Geometry: final body of the model. Coordinates: model frame, mm. A direction names the side the tool comes from. Give positions to 0.01 mm unless a question says otherwise; leave off trailing zeros. Order: outer loops, then holes, each group sorted by start corner. A loop starts at its lowest first (then second) coordinate and runs counter-clockwise, first axis right, second up. Notation, with made-up numbers: (59.5, 45.25) -> (93.5, 45.25) arc R26 ccw to (93.5, 80.25) -> close; hole circle Ø2 at (-21, 81). An arc over 180 degrees is marked (long way). One line per item, written item: value. Start each with the question number.
```python
from build123d import *

# Parameters (mm, degrees)
SKETCH17_R                     = 3.4
SKETCH17_W                     = 3.75
SKETCH17_H                     = 3.75
T_SLOT_PROFILES_3030_2_1_DEPTH = 400


with BuildPart() as part:
    # Sketch17 → T-slot profiles 3030_2(1) (new body)
    with BuildSketch(Plane(origin=(0, 0, 0), x_dir=(0, 0, -1), z_dir=(1, 0, 0))):
        with BuildLine():
            Line((-4.07, 5.6), (4.07, 5.6))
            Line((4.07, 5.6), (8.25, 9.78))
            Line((8.25, 9.78), (8.25, 13))
            Line((8.25, 13), (4.07, 13))
            Line((4.07, 13), (4.07, 15))
            Line((4.07, 15), (12.5, 15))
            ThreePointArc((12.5, 15), (14.267766953, 14.267766953), (15, 12.5))
            Line((15, 12.5), (15, 4.07))
            Line((15, 4.07), (13, 4.07))
            Line((13, 4.07), (13, 8.25))
            Line((13, 8.25), (9.78, 8.25))
            Line((9.78, 8.25), (5.6, 4.07))
            Line((5.6, 4.07), (5.6, -4.07))
            Line((5.6, -4.07), (9.78, -8.25))
            Line((9.78, -8.25), (13, -8.25))
            Line((13, -8.25), (13, -4.07))
            Line((13, -4.07), (15, -4.07))
            Line((15, -4.07), (15, -12.5))
            ThreePointArc((15, -12.5), (14.267766953, -14.267766953), (12.5, -15))
            Line((12.5, -15), (4.07, -15))
            Line((4.07, -15), (4.07, -13))
            Line((4.07, -13), (8.25, -13))
            Line((8.25, -13), (8.25, -9.78))
            Line((8.25, -9.78), (4.07, -5.6))
            Line((4.07, -5.6), (-4.07, -5.6))
            Line((-4.07, -5.6), (-8.25, -9.78))
            Line((-8.25, -9.78), (-8.25, -13))
            Line((-8.25, -13), (-4.07, -13))
            Line((-4.07, -13), (-4.07, -15))
            Line((-4.07, -15), (-12.5, -15))
            ThreePointArc((-12.5, -15), (-14.267766953, -14.267766953), (-15, -12.5))
            Line((-15, -12.5), (-15, -4.07))
            Line((-15, -4.07), (-13, -4.07))
            Line((-13, -4.07), (-13, -8.25))
            Line((-13, -8.25), (-9.78, -8.25))
            Line((-9.78, -8.25), (-5.6, -4.07))
            Line((-5.6, -4.07), (-5.6, 4.07))
            Line((-5.6, 4.07), (-9.78, 8.25))
            Line((-9.78, 8.25), (-13, 8.25))
            Line((-13, 8.25), (-13, 4.07))
            Line((-13, 4.07), (-15, 4.07))
            Line((-15, 4.07), (-15, 12.5))
            ThreePointArc((-15, 12.5), (-14.267766953, 14.267766953), (-12.5, 15))
            Line((-12.5, 15), (-4.07, 15))
            Line((-4.07, 15), (-4.07, 13))
            Line((-4.07, 13), (-8.25, 13))
            Line((-8.25, 13), (-8.25, 9.78))
            Line((-8.25, 9.78), (-4.07, 5.6))
        make_face()
        Circle(SKETCH17_R, mode=Mode.SUBTRACT)
        with Locations((11.625, 11.625)):
            Rectangle(SKETCH17_W, SKETCH17_H, mode=Mode.SUBTRACT)
        with Locations((11.625, -11.625)):
            Rectangle(SKETCH17_W, SKETCH17_H, mode=Mode.SUBTRACT)
        with Locations((-11.625, 11.625)):
            Rectangle(SKETCH17_W, SKETCH17_H, mode=Mode.SUBTRACT)
        with Locations((-11.625, -11.625)):
            Rectangle(SKETCH17_W, SKETCH17_H, mode=Mode.SUBTRACT)
    extrude(amount=T_SLOT_PROFILES_3030_2_1_DEPTH)


solid = part.part
```
1. Draft query along Y for faces 6 (the flat face through (197, -15, 8)), 7 (the flat face through (400, -3, 2)), 8 (the flat face through (197, 0, 5.6)). Return one class per face: pulls with the +Y half, pulls with the -Y half, needs draft (parallel to the pull), parting line crosses it, or undercut.
2. Cut plane C-C, the plane x = 92. State how many separate pieces and enclosed holes the cut face has, then the cut area to 3 significant figures.
3. Cut plane A-A, the plane z = 0. Return loops of the section in (x, y), then the cut area to 3 significant figures.
4. Pin query (flat end, axial travel): P1, Ø0.6, axis at x = 110, z = -14, coming from the +Y side; P2, Ø1.5, axis at x = 199, y = 1, coming from the -Z side; P3, Ø2.5, axis at x = 228, z = 1.5, coming from the -Y side. Return the tip coordinate at first contact, or that it passes through.
5. Access query for faces 1 (the flat face through (197, 8, 15)), 2 (the flat face through (197, 8, -15)), 3 (the flat face through (197, 0, -5.6)), 4 (the flat face through (197, -5.6, 0)), 5 (the flat face through (197, 5.6, 0)). Directions: +Z, -Z, +X, -X, +Y, -Y. A direction counts if a zero-diameter tool reaches every point of the face in a straight line with its end or side. Return the directions, or none.
6. Material intervals for L1, parallel to Z at x = 153, y = 10.5; L2, parallel to Y at x = 142, z = 0; L3, parallel to Y at x = 48.5, z = -5, sorted ascending. Write a range as [from, to].
Answers follow:
1. face 6: pulls with the -Y half
1. face 7: needs draft
1. face 8: undercut
2. separate pieces: 1
2. enclosed holes: 5
2. area: 318 mm²
3. outline: (0, -5.6) -> (400, -5.6) -> (400, -3.4) -> (0, -3.4) -> close; (0, 3.4) -> (400, 3.4) -> (400, 5.6) -> (0, 5.6) -> close
3. area: 1,760 mm²
4. P1: stops at y = 14.69
4. P2: stops at z = -5.6
4. P3: stops at y = -5.6
5. face 1: +Z, +X, -X, +Y, -Y
5. face 2: -Z, +X, -X, +Y, -Y
5. face 3: -Z, +X, -X
5. face 4: +X, -X, -Y
5. face 5: +X, -X, +Y
6. L1: z = [-15, -13.5], [-9.75, -8.25], [8.25, 9.75], [13.5, 15]
6. L2: y = [-5.6, -3.4], [3.4, 5.6]
6. L3: y = [-15, -13], [-6.53, 6.53], [13, 15]
